```python
from build123d import *

# Parameters (mm, degrees)
F1_DEPTH = 3.175
F2_W     = 254
F2_H     = 25.4
F3_DEPTH = 3.176


with BuildPart() as f1:
    # F0 (on Top) → F1 (new body)
    with BuildSketch(Plane.XY):
        Polygon((-276.225, -287.3375), (276.225, -287.3375), (276.225, -228.6), (279.4, -228.6), (279.4, -152.4), (276.225, -152.4), (276.225, -38.1), (279.4, -38.1), (279.4, 38.1), (276.225, 38.1), (276.225, 152.4), (279.4, 152.4), (279.4, 228.6), (276.225, 228.6), (276.225, 287.3375), (-276.225, 287.3375), (-276.225, 228.6), (-279.4, 228.6), (-279.4, 152.4), (-276.225, 152.4), (-276.225, 38.1), (-279.4, 38.1), (-279.4, -38.1), (-276.225, -38.1), (-276.225, -152.4), (-279.4, -152.4), (-279.4, -228.6), (-276.225, -228.6), align=None)
    extrude(amount=F1_DEPTH)

    # F2 (on face) → F3 (cut, through all)
    with BuildSketch(Plane.XY.offset(3.175)):
        with Locations((0, -249.2375)):
            Rectangle(F2_W, F2_H)
    extrude(amount=-F3_DEPTH, mode=Mode.SUBTRACT)


solid = f1.part
```
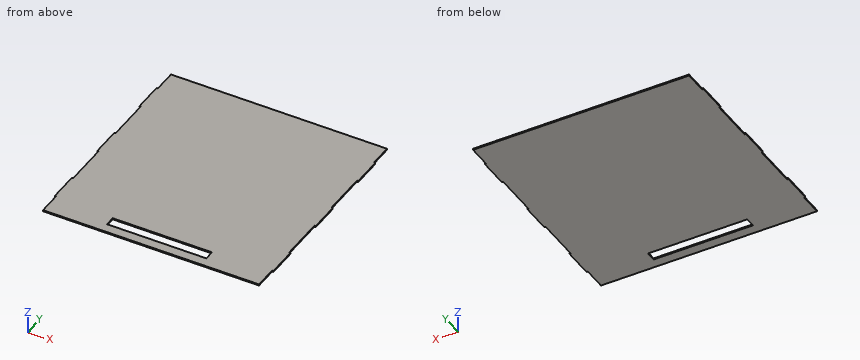
Design review of the part built by this model. Coordinates are the model's own, in mm. Give positions to 0.01 mm unless a question says otherwise; leave off trailing zeros. Order: outer loops, then holes, each group sorted by start corner. A loop starts at its lowest first (then second) coordinate and runs counter-clockwise, first axis right, second up. Notation, with made-up numbers: M 43.5,19.5 L 99.5,19.5 A18 cw 99.5,37.5 Z; hole C 88.5,48 d9. An arc over 180 degrees is marked long. One line per question, with ' | ' between items. Start each with the question number.
Q1. For L1, parallel to Y at x = -117, z = 1.9; L2, parallel to X at y = -80, z = 2.25 (3 decimals), list the stretches that pass through material, from the lowest coordinate up. Write a range as [from, to].
Q2. For pin 1 Ø1.6 at (x, z) = (-277.5, 2.5) entering from +Y; pin 2 Ø1.6 at (y, z) = (255.5, 2) entering from +X (3 decimals); pin 3 Ø1.6 at (x, z) = (-278, 1.5) entering from -Y, all flat-tipped, find the tip position at first contact; note any pin that passes through.
Q3. We need section A-A (x = -95.5). Write out the cut boundary in (y, z) (1 decimal).
Returned:
1) L1: [-287.34, -261.94], [-236.54, 287.34] | L2: [-276.225, 276.225]
2) pin 1: y = 228.6 | pin 2: x = 276.225 | pin 3: y = -228.6
3) outline: M -287.3,0 L -261.9,0 L -261.9,3.2 L -287.3,3.2 Z; M -236.5,0 L 287.3,0 L 287.3,3.2 L -236.5,3.2 Z
